Source: CAD feature listing. Evaluate the final solid. Frame: model axes, mm. Round coordinates to 2 decimals unless told otherwise and drop trailing zeros. Order: outer loops, then holes, each group sorted by start corner. A loop starts at its lowest first (then second) coordinate and runs counter-clockwise, first axis right, second up. Notation, with made-up numbers: (-10.5, -38) -> (46.5, -38) arc R36 ccw to (46.5, -4) -> close; hole circle Ø1 at (83.5, 27.5). An arc over 180 degrees is marked (long way). One line per item, written item: value. Start each with the question number.
1) Section D-D (x = 0). Return the cut outline in (y, z), and give its area (3 significant figures).
2) Section B-B (z = 0.35). Return the cut outline in (x, y).
3) Section A-A (y = -5). Return the cut outline in (x, z), and give its area (3 significant figures).
4) Section C-C (x = 3.5). Return the cut outline in (y, z), and give its area (3 significant figures).
5) Mould query, pull axis X, two halves, no side actions, for faces 1 (the face through (0.179, 5.397, 0.394)), 2 (the face through (-0.165, 3.796, 0.394)), 3 (the face through (2.2, -3.3, 0.8)). Classes: pulls with the +X half, pulls with the -X half, needs draft (parallel to the pull), parting line crosses it, or undercut.
6) Ray query, L1, parallel to Y at x = 1, z = 0.1; L2, parallel to Y at x = -1.25, z = 0.2; L3, parallel to Y at x = -3, z = 0.3. Return the intervals inside material, ascending.
7) Pin query (flat end, axial travel): P1, Ø2, axis at x = 1, y = -3, coming from the -Z side. Return the tip coordinate at first contact, or that it passes through.
```python
from build123d import *

# Parameters (mm, degrees)
BOSS_EXTRUDE1_DEPTH = 0.8
SKETCH2_R           = 0.5
CUT_EXTRUDE1_DEPTH  = 9.478207358
DELETEFACE1_DEPTH   = 0.8
CUT_EXTRUDE2_DEPTH  = 9.478207358


# Read off the part's stored shape, not the designer's step: DeleteFace1
with BuildPart() as part:
    # Sketch1 → Boss-Extrude1 (new body)
    with BuildSketch(Plane.XY):
        with BuildLine():
            Line((-2.5, -4.209772229), (-2.5, -6.3))
            ThreePointArc((-2.5, -6.3), (-2.353553391, -6.653553391), (-2, -6.8))
            Line((-2, -6.8), (-0.15, -6.8))
            Line((-0.15, -6.8), (-0.15, -3.79703832))
            ThreePointArc((-0.15, -3.79703832), (0, 3.8), (0.15, -3.79703832))
            Line((0.15, -3.79703832), (0.15, -6.8))
            Line((0.15, -6.8), (2, -6.8))
            ThreePointArc((2, -6.8), (2.353553391, -6.653553391), (2.5, -6.3))
            Line((2.5, -6.3), (2.5, -4.209772229))
            ThreePointArc((2.5, -4.209772229), (2.560475464, -3.971406581), (2.727272727, -3.790702026))
            ThreePointArc((2.727272727, -3.790702026), (0, 5.4), (-2.727272727, -3.790702026))
            ThreePointArc((-2.727272727, -3.790702026), (-2.560475464, -3.971406581), (-2.5, -4.209772229))
        make_face()
    extrude(amount=BOSS_EXTRUDE1_DEPTH)

    # Sketch2 → Cut-Extrude1 (cut, through all)
    with BuildSketch(Plane(origin=(0, 0, 0), x_dir=(-1, 0, 0), z_dir=(0, 0, -1))):
        with Locations((-0.6, -5.3)):
            Circle(SKETCH2_R)
        with Locations((0.6, -5.3)):
            Circle(SKETCH2_R)
    extrude(amount=-CUT_EXTRUDE1_DEPTH, mode=Mode.SUBTRACT)

    # DeleteFace1 outline → DeleteFace1 (add)
    with BuildSketch(Plane.XY):
        with BuildLine():
            Line((-0.15, -5.517944947), (-0.15, -5.082055053))
            ThreePointArc((-0.15, -5.082055053), (-1.1, -5.3), (-0.15, -5.517944947))
        make_face()
        with BuildLine():
            Line((0.15, -5.082055053), (0.15, -5.517944947))
            ThreePointArc((0.15, -5.517944947), (1.1, -5.3), (0.15, -5.082055053))
        make_face()
    extrude(amount=DELETEFACE1_DEPTH)

    # Sketch3 → Cut-Extrude2 (cut, through all)
    with BuildSketch(Plane(origin=(0, 0, 0), x_dir=(-1, 0, 0), z_dir=(0, 0, -1))):
        with BuildLine():
            Line((-0.6, -4.8), (0.6, -4.8))
            ThreePointArc((0.6, -4.8), (1.1, -5.3), (0.6, -5.8))
            Line((0.6, -5.8), (-0.6, -5.8))
            ThreePointArc((-0.6, -5.8), (-1.1, -5.3), (-0.6, -4.8))
        make_face()
    extrude(amount=-CUT_EXTRUDE2_DEPTH, mode=Mode.SUBTRACT)


solid = part.part
```
Findings:
1. outline: (3.8, 0) -> (5.4, 0) -> (5.4, 0.8) -> (3.8, 0.8) -> close
1. area: 1.28 mm2
2. outline: (-2.73, -3.79) arc R0.5 cw to (-2.5, -4.21) -> (-2.5, -6.3) arc R0.5 ccw to (-2, -6.8) -> (-0.15, -6.8) -> (-0.15, -5.8) -> (-0.6, -5.8) arc R0.5 cw to (-0.6, -4.8) -> (-0.15, -4.8) -> (-0.15, -3.8) arc R3.8 cw (long way) to (0.15, -3.8) -> (0.15, -4.8) -> (0.6, -4.8) arc R0.5 cw to (0.6, -5.8) -> (0.15, -5.8) -> (0.15, -6.8) -> (2, -6.8) arc R0.5 ccw to (2.5, -6.3) -> (2.5, -4.21) arc R0.5 cw to (2.73, -3.79) arc R5 ccw (long way) to start
3. outline: (-2.5, 0) -> (-1, 0) -> (-1, 0.8) -> (-2.5, 0.8) -> close; (1, 0) -> (2.5, 0) -> (2.5, 0.8) -> (1, 0.8) -> close
3. area: 2.40 mm2
4. outline: (-3.17, 0) -> (-1.48, 0) -> (-1.48, 0.8) -> (-3.17, 0.8) -> close; (1.48, 0) -> (3.97, 0) -> (3.97, 0.8) -> (1.48, 0.8) -> close
4. area: 3.35 mm2
5. face 1: parting line crosses it
5. face 2: undercut
5. face 3: needs draft
6. L1: -6.8 to -5.6, -5 to -3.67, 3.67 to 5.3
6. L2: -6.8 to -3.59, 3.59 to 5.24
6. L3: -3.6 to -2.33, 2.33 to 4.4
7. P1: z = 0
